```python
from build123d import *

# Parameters (mm, degrees)
F1_DEPTH = 25.4
F2_R     = 5.07999


# Not quite as in the source:
# - a fillet or chamfer is up to 0.001 mm smaller than in the source, because OpenCascade refuses the exact size


with BuildPart() as f1:
    # F0 (on Front) → F1 (new body)
    with BuildSketch(Plane.XZ):
        Polygon((25.4, 0), (0, 0), (0, -25.4), (5.08, -25.4), (5.08, -5.08), (20.32, -5.08), (20.32, -25.4), (25.4, -25.4), align=None)
    extrude(amount=F1_DEPTH)

    # F2 (radius 5.08 in the source; OpenCascade refuses exactly that, so slightly less here)
    f2_edges = [f1.edges().sort_by_distance(p)[0] for p in [
        (0, -12.7, 0),
        (12.7, -25.4, 0),
        (25.4, -12.7, 0),
        (12.7, 0, 0),
        (0, -25.4, -12.7),
        (0, 0, -12.7),
        (25.4, 0, -12.7),
        (25.4, -25.4, -12.7),
        (0, -12.7, -25.4),
        (25.4, -12.7, -25.4),
    ]]
    fillet(f2_edges, radius=F2_R)


solid = f1.part
```
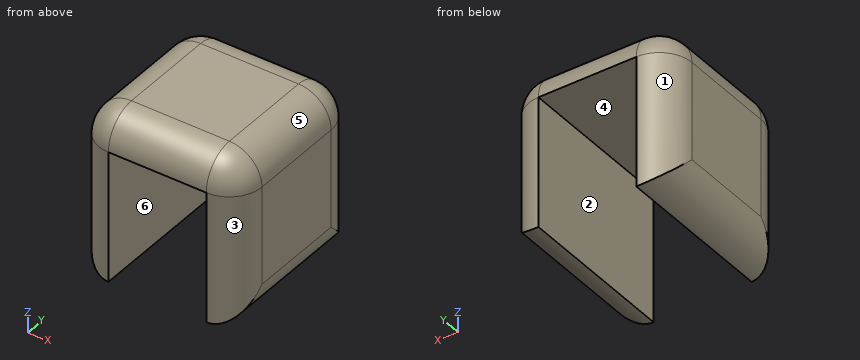
Geometry check sheet. Reference: the model listing, model coordinates, mm. Face numbers are marked on the shaded views. A direction names the side the tool comes from. Give positions to 0.01 mm unless a question says otherwise; leave off trailing zeros. Write each loop counter-clockwise with the first axis right and the second up, starting at its lowest first coordinate (ties: lowest second). Pieces come first, ordered by that corner, then holes.
1) Section check D-D, the plane x = 21. Record the boundary of the cut face in (y, z), and give its area (3 significant figures).
2) Section check C-C, the plane z = -4.5. Record the boundary of the cut face in (x, y), and give its area (3 significant figures).
3) Access from +Z, -Z, +X, -X, +Y, -Y to the whole of each face (thin tool, end or side, straight path). Record for the marked faces 5 and 6.
4) Material ranges on L1, parallel to X at y = -18.75, z = -19.25; L2, parallel to Z at x = 9, y = -16.25; L3, parallel to X at y = -2.75, z = -14.5, recorded low to high.
5) Gauge pin test, flat ends, axial feed: pin 1 (1.5 mm diameter, centred on x = 3.5, y = -5, fed in from -Z); pin 2 (2 mm diameter, centred on x = 6.5, y = -21.5, fed in from +Z); pin 3 (1.5 mm diameter, centred on x = 2.5, y = -16.5, fed in from +Z). Record the tip position at first contact, or that the pin passes through.
6) Release check for a two-part mould opening along X. For the marked faces 1, 2, 3 and 4 record: pulls with the +X half, pulls with the -X half, needs draft (parallel to the pull), parting line crosses it, or undercut.
Computed:
1. outline: (-25.35, -25.35) - (-0.05, -25.35) - (-0.05, -5.08) arc R5.03 ccw to (-5.08, -0.05) - (-20.32, -0.05) arc R5.03 ccw to (-25.35, -5.08) - close
1. area: 630 mm2
2. outline: (0.03, -20.32) arc R5.05 ccw to (5.08, -25.37) - (20.32, -25.37) arc R5.05 ccw to (25.37, -20.32) - (25.37, -5.08) arc R5.05 ccw to (20.32, -0.03) - (5.08, -0.03) arc R5.05 ccw to (0.03, -5.08) - close
2. area: 620 mm2
3. face 5: +Z, +X, +Y, -Y
3. face 6: -Z, +Y, -Y
4. L1: x = 0 to 5.08, 20.32 to 25.4
4. L2: z = -5.08 to 0
4. L3: x = 0.57 to 5.08, 20.32 to 24.83
5. pin 1: stops at z = -25.33
5. pin 2: stops at z = 0
5. pin 3: stops at z = -0.34
6. face 1: pulls with the -X half
6. face 2: undercut
6. face 3: pulls with the +X half
6. face 4: undercut
